For this review, take the finished solid that the model builds, in its own axes (mm). A direction names the side the tool comes from. Round coordinates to 2 decimals unless told otherwise and drop trailing zeros. Loops run counter-clockwise (first coordinate to the right, second up) from the corner with the lowest first, then second, coordinate; pieces in that order, holes last.
1. Draft analysis for pull direction Z (two halves, no side actions). For faces 1 (the cylindrical face through (-15.023, 13.465, -15.38)), 2 (the cylindrical face through (-24.43, 12.06, -0.25)), 3 (the cylindrical face through (16.915, 6.938, 1.084)), state which applies: released by +Z, released by -Z, zero draft, split by the parting line, or undercut.
2. Consider section B-B on y = 9.25. State the section outline as (x, z) points, then the cut area to 3 significant figures.
3. Clearance check with flat-ended pins moving along their axes: pin 1 Ø8 at (y, z) = (11, -19.5) entering from +X; pin 2 Ø6 at (x, z) = (-1.5, 9.5) entering from -Y; pin 3 Ø2.5 at (x, z) = (19, -0.5) entering from +Y; pin 4 Ø1.5 at (x, y) = (-19.5, 3) entering from +Z. State where each tip first meets the part, or that it passes through.
4. Consider section D-D on y = 13.25. State the section outline as (x, z) points, then the cut area to 3 significant figures.
5. To check wall thickness, follow line 1 along X through (y, z) = (11, 0); line 2 along Z through (x, y) = (-19.5, 3); line 3 along X through (y, z) = (15, 1). State the ranges of each line that lie inside material, in increasing order.
6. Consider section C-C on y = 3. State how many separate pieces and enclosed holes the cut face has, then the cut area to 3 significant figures.
7. Tool access review of faces 4 (the cylindrical face through (-0.356, 12.059, 24.304)), 5 (the cylindrical face through (30.77, 4.25, -7.85)), 6 (the cylindrical face through (-20.43, 6.938, -1.865)), 7 (the flat face through (0, 1, -19)): name each direction out of +Z, -Z, +X, -X, +Y, -Y from which nothing blocks a thin tool from reaching the whole face with its end or side.
from build123d import *

# Parameters (mm, degrees)
SKETCH2_R           = 35
SKETCH2_R_2         = 21
SKETCH2_R_3         = 2.65
BOSS_EXTRUDE6_DEPTH = 8
SKETCH3_R           = 21.5
SKETCH3_R_2         = 14.25
BOSS_EXTRUDE7_DEPTH = 16
FILLET1_R           = 3
SKETCH4_R           = 2.35
CUT_EXTRUDE1_DEPTH  = 15
BOSS_EXTRUDE9_REACH = 54.019
SKETCH7_R           = 2.35
CHAMFER1_SIZE       = 0.6


with BuildPart() as part:
    # Sketch2 → Boss-Extrude6 (new body)
    with BuildSketch(Plane(origin=(0, 0, 0), x_dir=(1, 0, 0), z_dir=(0, 1, 0))):
        with Locations(Location((0, 0, 0), (0, 0, 270))):
            Circle(SKETCH2_R)
        with Locations(Location((0, 0, 0), (0, 0, 270))):
            Circle(SKETCH2_R_2, mode=Mode.SUBTRACT)
        with Locations(Location((0, 30, 0), (0, 0, 270))):
            Circle(SKETCH2_R_3, mode=Mode.SUBTRACT)
        with Locations(Location((28.531695489, 9.270509831, 0), (0, 0, 270))):
            Circle(SKETCH2_R_3, mode=Mode.SUBTRACT)
        with Locations(Location((17.633557569, -24.270509831, 0), (0, 0, 270))):
            Circle(SKETCH2_R_3, mode=Mode.SUBTRACT)
        with Locations(Location((-17.633557569, -24.270509831, 0), (0, 0, 270))):
            Circle(SKETCH2_R_3, mode=Mode.SUBTRACT)
        with Locations(Location((-28.531695489, 9.270509831, 0), (0, 0, 270))):
            Circle(SKETCH2_R_3, mode=Mode.SUBTRACT)
    extrude(amount=BOSS_EXTRUDE6_DEPTH)

    # Sketch3 → Boss-Extrude7 (add)
    with BuildSketch(Plane(origin=(0, 0, 0), x_dir=(1, 0, 0), z_dir=(0, 1, 0))):
        with Locations(Location((0, 0, 0), (0, 0, 270))):
            Circle(SKETCH3_R)
        with Locations(Location((0, 0, 0), (0, 0, 270))):
            Circle(SKETCH3_R_2, mode=Mode.SUBTRACT)
    extrude(amount=BOSS_EXTRUDE7_DEPTH)

    # Fillet1
    fillet1_edges = [part.edges().sort_by_distance(p)[0] for p in [
        (0, 8, -21.5),
    ]]
    fillet(fillet1_edges, radius=FILLET1_R)

    # Sketch4 → Cut-Extrude1 (cut)
    with BuildSketch(Plane(origin=(0, 16, 0), x_dir=(1, 0, 0), z_dir=(0, 1, 0))):
        with Locations(Location((0, 19, 0), (0, 0, 270))):
            Circle(SKETCH4_R)
        with Locations(Location((19, 0, 0), (0, 0, 270))):
            Circle(SKETCH4_R)
        with Locations(Location((0, -19, 0), (0, 0, 270))):
            Circle(SKETCH4_R)
        with Locations(Location((-19, 0, 0), (0, 0, 270))):
            Circle(SKETCH4_R)
    extrude(amount=-CUT_EXTRUDE1_DEPTH, mode=Mode.SUBTRACT)

    # Boss-Extrude9: up to this face of the body (flat: up to its plane)
    boss_extrude9_end = Plane(part.part.faces().sort_by_distance((0, 8, -25.489949494))[0])
    # Sketch7 → Boss-Extrude9 (add, up to the picked face)
    with BuildSketch(Plane(origin=(0, 16, 0), x_dir=(1, 0, 0), z_dir=(0, 1, 0)), mode=Mode.PRIVATE) as boss_extrude9_sk1:
        with BuildLine():
            Line((-4.477866444, 16.072336749), (4.398028303, 15.953715863))
            ThreePointArc((4.398028303, 15.953715863), (0.071493082, 24.349522291), (-4.477866444, 16.072336749))
        make_face()
        with Locations(Location((0, 19, 0), (0, 0, 270))):
            Circle(SKETCH7_R, mode=Mode.SUBTRACT)
    boss_extrude9_tool1 = split(extrude(boss_extrude9_sk1.sketch, amount=-BOSS_EXTRUDE9_REACH, mode=Mode.PRIVATE), bisect_by=boss_extrude9_end, keep=Keep.BOTH, mode=Mode.PRIVATE)
    # Sketch7 → Boss-Extrude9 (add, up to the picked face)
    with BuildSketch(Plane(origin=(0, 16, 0), x_dir=(1, 0, 0), z_dir=(0, 1, 0)), mode=Mode.PRIVATE) as boss_extrude9_sk2:
        with BuildLine():
            Line((15.946789092, 4.395782427), (15.828168206, -4.48011232))
            ThreePointArc((15.828168206, -4.48011232), (24.223974633, -0.153577099), (15.946789092, 4.395782427))
        make_face()
        with Locations((18.874452343, -0.082084016)):
            Circle(SKETCH7_R, mode=Mode.SUBTRACT)
    boss_extrude9_tool2 = split(extrude(boss_extrude9_sk2.sketch, amount=-BOSS_EXTRUDE9_REACH, mode=Mode.PRIVATE), bisect_by=boss_extrude9_end, keep=Keep.BOTH, mode=Mode.PRIVATE)
    # Sketch7 → Boss-Extrude9 (add, up to the picked face)
    with BuildSketch(Plane(origin=(0, 16, 0), x_dir=(1, 0, 0), z_dir=(0, 1, 0)), mode=Mode.PRIVATE) as boss_extrude9_sk3:
        with BuildLine():
            Line((4.27023477, -16.028873108), (-4.605659977, -15.910252222))
            ThreePointArc((-4.605659977, -15.910252222), (-0.279124756, -24.30605865), (4.27023477, -16.028873108))
        make_face()
        with Locations((-0.207631674, -18.956536359)):
            Circle(SKETCH7_R, mode=Mode.SUBTRACT)
    boss_extrude9_tool3 = split(extrude(boss_extrude9_sk3.sketch, amount=-BOSS_EXTRUDE9_REACH, mode=Mode.PRIVATE), bisect_by=boss_extrude9_end, keep=Keep.BOTH, mode=Mode.PRIVATE)
    # Sketch7 → Boss-Extrude9 (add, up to the picked face)
    with BuildSketch(Plane(origin=(0, 16, 0), x_dir=(1, 0, 0), z_dir=(0, 1, 0)), mode=Mode.PRIVATE) as boss_extrude9_sk4:
        with BuildLine():
            Line((-16.154420765, -4.352318786), (-16.035799879, 4.523575961))
            ThreePointArc((-16.035799879, 4.523575961), (-24.431606307, 0.19704074), (-16.154420765, -4.352318786))
        make_face()
        with Locations((-19.082084016, 0.125547657)):
            Circle(SKETCH7_R, mode=Mode.SUBTRACT)
    boss_extrude9_tool4 = split(extrude(boss_extrude9_sk4.sketch, amount=-BOSS_EXTRUDE9_REACH, mode=Mode.PRIVATE), bisect_by=boss_extrude9_end, keep=Keep.BOTH, mode=Mode.PRIVATE)
    add(boss_extrude9_tool1.solids().sort_by(Axis((0.069676, 16, -24.213524), (0, -1, 0)))[0])
    add(boss_extrude9_tool2.solids().sort_by(Axis((16.023477, 16, 0.043982), (0, -1, 0)))[0])
    add(boss_extrude9_tool3.solids().sort_by(Axis((-0.277307, 16, 24.170061), (0, -1, 0)))[0])
    add(boss_extrude9_tool4.solids().sort_by(Axis((-16.231108, 16, -0.087446), (0, -1, 0)))[0])

    # Chamfer1
    chamfer1_edges = [part.edges().sort_by_distance(p)[0] for p in [
        (28.531695489, 0, -11.920509831),
        (17.633557569, 0, 21.620509831),
        (0, 0, -35),
        (-17.633557569, 0, 21.620509831),
        (-28.531695489, 0, -11.920509831),
        (0, 0, -14.25),
        (0, 0, -32.65),
    ]]
    chamfer(chamfer1_edges, length=CHAMFER1_SIZE)


solid = part.part
Resolved:
1. face 1: released by -Z
1. face 2: split by the parting line
1. face 3: undercut
2. outline: (-21.58, 4.61) arc R5.35 ccw to (-21.51, -4.89) arc R22.06 ccw to (-4.7, -21.56) arc R5.35 ccw to (4.7, -21.56) arc R22.06 ccw to (21.59, -4.52) arc R5.35 ccw to (21.55, 4.71) arc R22.06 ccw to (4.44, 21.61) arc R5.35 ccw to (-4.91, 21.51) arc R22.06 ccw to start; hole (-21.01, 1.22) arc R2.35 ccw to (-17.08, -1.35) arc R2.35 ccw to start; hole circle Ø28.5 at (0, 0); hole circle Ø4.7 at (0, -19); hole (-0.58, 21.28) arc R2.35 ccw to (0.38, 16.68) arc R2.35 ccw to start; hole (17.65, -1.92) arc R2.35 ccw to (20.22, 2.01) arc R2.35 ccw to start
2. area: 886 mm2
3. pin 1: stops at x = 30.67
3. pin 2: passes through
3. pin 3: stops at y = 1
3. pin 4: stops at z = 29.55
4. outline: (-20.94, 4.89) arc R5.35 ccw to (-20.87, -5.17) arc R21.5 ccw to (-5, -20.91) arc R5.35 ccw to (5, -20.91) arc R21.5 ccw to (20.95, -4.85) arc R5.35 ccw to (20.9, 5.03) arc R21.5 ccw to (4.75, 20.97) arc R5.35 ccw to (-5.21, 20.86) arc R21.5 ccw to start; hole (-21.01, 1.22) arc R2.35 ccw to (-17.08, -1.35) arc R2.35 ccw to start; hole circle Ø28.5 at (0, 0); hole circle Ø4.7 at (0, -19); hole (-0.58, 21.28) arc R2.35 ccw to (0.38, 16.68) arc R2.35 ccw to start; hole (17.65, -1.92) arc R2.35 ccw to (20.22, 2.01) arc R2.35 ccw to start
4. area: 831 mm2
5. line 1: x = -24.43 to -21.35, -16.74 to -14.25, 14.25 to 16.65, 21.22 to 24.22
5. line 2: z = -29.06 to -2.3, 2.3 to 22.39, 26.15 to 29.06
5. line 3: x = -24.31 to -21.13, -17.02 to -14.21, 14.21 to 16.87, 21.04 to 24.15
6. separate pieces: 1
6. enclosed holes: 10
6. area: 3,030 mm2
7. face 4: +Z, +Y
7. face 5: +Y, -Y
7. face 6: none
7. face 7: +Y
